Can you work these out from the model? Positions are in its coordinate system, mm. A direction names the side the tool comes from. Coordinates: 2 decimals unless noted, no trailing zeros. Loops run counter-clockwise (first coordinate to the right, second up) from the corner with the lowest first, then second, coordinate; pieces in that order, holes last.
Autodesk Inventor part; units mm, degrees
ref_plane "YZ Plane" through (0, 0, 0) normal (1, 0, 0) x (0, 1, 0)
ref_plane "XZ Plane" through (0, 0, 0) normal (0, 1, 0) x (-1, 0, 0)
ref_plane "XY Plane" through (0, 0, 0) normal (0, 0, 1) x (1, 0, 0)
sketch "Sketch1" plane through (0, 0, 0) normal (0, 1, 0) x (-1, 0, 0)
  line L0 (0, 0) -> (0, 5) construction
  line L1 (-3.3166, 5) -> (3.3166, 5)
  line L2 (-8.6998, 0) -> (12.7628, 0) construction
  line L3 (-3.3166, -5) -> (3.3166, -5)
  arc A0 (-3.3166, 5) -> (-3.3166, -5) centre (0, 0) ccw
  arc A1 (3.3166, -5) -> (3.3166, 5) centre (0, 0) ccw
  dimension "d1" = 5
extrude "Extrusion1" add sketch "Sketch1" along normal blind 15
sketch "Sketch2" plane through (0, 15, 0) normal (0, 1, 0) x (1, 0, 0)
  arc A0 (-3.3166, 5) -> (-3.3166, -5) centre (0, 0) ccw
  line L0 (-6, -5) -> (6, -5)
  line L1 (6, -5) -> (6, 5)
  line L2 (6, 5) -> (-6, 5)
  line L3 (-6, 5) -> (-6, -5)
  line L4 (-6, -5) -> (6, 5) construction
  line L5 (6, -5) -> (-6, 5) construction
extrude "Extrusion2" add sketch "Sketch2" along normal blind 9
sketch "Sketch3" plane through (0, 24, 0) normal (0, 1, 0) x (1, 0, 0)
  line L0 (-6, 5) -> (-6, -5)
  arc A0 (-1.118, 1) -> (1.118, 1) centre (0, 0) ccw
  line L1 (0, -1.5) -> (0, 1) construction
  line L2 (-1.118, 1) -> (1.118, 1)
  dimension "d6" = 3
  dimension "d7" = 2.5
extrude "Extrusion3" add sketch "Sketch3" along normal blind 9.27
sketch "Sketch5" plane through (0, 0, 0) normal (0, -1, 0) x (1, 0, 0)
  line L0 (0, 0) -> (0, 3.5) construction
  line L1 (0, 3.5) -> (0.75, 3.5)
  line L2 (0, 3.5) -> (-0.75, 3.5)
  line L3 (0.75, 3.5) -> (0.75, 3.2)
  line L4 (0.75, 3.2) -> (-0.75, 3.2)
  line L5 (-0.75, 3.2) -> (-0.75, 3.5)
  line L6 (7.0613, 0) -> (-6.7326, 0) construction
  line L7 (-0.75, -3.2) -> (-0.75, -3.5)
  line L8 (0.75, -3.2) -> (-0.75, -3.2)
  line L9 (0.75, -3.5) -> (0.75, -3.2)
  line L10 (0, 0) -> (0, -3.5) construction
  line L11 (0, -3.5) -> (0.75, -3.5)
  line L12 (0, -3.5) -> (-0.75, -3.5)
  dimension "d14" = 3.5
  dimension "d15" = 0.75
  dimension "d16" = 0.3
extrude "Extrusion4" add sketch "Sketch5" along normal blind 1.5
sketch "Sketch6" plane through (0, 0, 0) normal (0, -1, 0) x (1, 0, 0)
  arc A0 (3.3166, -5) -> (3.3166, 5) centre (0, 0) ccw
  circle A1 centre (0, 0) radius 2.5
  dimension "d19" = 5
extrude "Extrusion5" add sketch "Sketch6" along normal blind 2
properties part number "motor pololu"
Item 1: Suppose I cut it at D-D, the plane z = -4.5. Please give me the cut outline in (x, y).
Results are:
outline: (-6, 15) - (-3.97, 15) - (-3.97, 0) - (3.97, 0) - (3.97, 15) - (6, 15) - (6, 24) - (-6, 24) - close
Item 2: On a 3-axis mill with a long thin cutter (end or side, diameter ignored), from which of +Z, -Z, +X, -X, +Y, -Y can I reach the whole of each face in a straight line? I mean faces 1 (the face through (6, 7, 0)), 2 (the face through (-5.8, 15, -2.2)), 3 (the face through (0, 29, -1)), 4 (the face through (0, 28.6, 1.5)), 5 (the face through (0, -1, 3.2)). Say none if no direction works.
Results are:
face 1: +X, -Y
face 2: -X, -Y
face 3: -Z, +X, -X, +Y
face 4: +Y
face 5: +X, -X, -Y
Item 3: We'd pull the mould along Z, two halves only. Please class faces 6 (the face through (0, -1, -3.2)), 7 (the face through (-6, 7, 0)), 8 (the face through (0, -1, 3.5)), 9 (the face through (-0.54, -0.99, 2.44)): +Z half, -Z half, draft (parallel to the pull), parting line (faces both ways), or undercut.
Results are:
face 6: undercut
face 7: parting line
face 8: +Z half
face 9: undercut
Item 4: Suppose I cut it at B-B, the plane x = 0. Please give me the cut outline in (y, z), plus the area to 3 significant figures.
Results are:
outline: (-2, -2.5) - (0, -2.5) - (0, -3.2) - (-1.5, -3.2) - (-1.5, -3.5) - (0, -3.5) - (0, -5) - (24, -5) - (24, -1) - (33.27, -1) - (33.27, 1.5) - (24, 1.5) - (24, 5) - (0, 5) - (0, 3.5) - (-1.5, 3.5) - (-1.5, 3.2) - (0, 3.2) - (0, 2.5) - (-2, 2.5) - close
area: 274 mm2
Item 5: I'm going to push flat-ended pins straight in: P1, Ø3, axis at y = 10, z = 4, coming from the -X side; P2, Ø2, axis at x = 5, z = 2, coming from the -Y side; P3, Ø3, axis at x = 3, z = 1.5, coming from the +Y side. Where does each tip first touch, or does it pass through?
Results are:
P1: stops at x = -5.45
P2: stops at y = 0
P3: stops at y = 24
Item 6: I need wall thicknesses on line 1 along Y through (x, z) = (-3, 0.75); line 2 along Y through (x, z) = (4.75, -4.5); line 3 along X through (y, z) = (10, -2.5). Which ranges of each line are inside material? Lowest first, please.
Results are:
line 1: y = 0 to 24
line 2: y = 15 to 24
line 3: x = -5.45 to 5.45
Item 7: Suppose I cut it at C-C, the plane y = 27. Please give me the cut outline in (x, z).
Results are:
outline: (-1.12, -1) - (1.12, -1) arc R1.5 ccw (long way) to start
